from build123d import *

# Parameters (mm, degrees)
ESQUISSE1_R        = 5
ESQUISSE1_R_2      = 2.877506478
ESQUISSE1_R_3      = 3.063484505
ESQUISSE1_R_4      = 2.684325632
ESQUISSE1_R_5      = 0.5
BOSS_EXTRU_1_DEPTH = 3


with BuildPart() as part:
    # Esquisse1 → Boss.-Extru.1 (new body)
    with BuildSketch(Plane.XY):
        with BuildLine():
            Line((6, -6.708203932), (6, 0))
            Line((6, 0), (9, 0))
            Line((9, 0), (9.959071707, 27.096179922))
            ThreePointArc((9.959071707, 27.096179922), (0, 38), (-9.959071707, 27.096179922))
            Line((-9.959071707, 27.096179922), (-9, 0))
            Line((-9, 0), (-6, 0))
            Line((-6, 0), (-6, -6.708203932))
            ThreePointArc((-6, -6.708203932), (0, -9), (6, -6.708203932))
        make_face()
        Circle(ESQUISSE1_R, mode=Mode.SUBTRACT)
        with Locations((-4.874230419, 15.048067775)):
            Circle(ESQUISSE1_R_2, mode=Mode.SUBTRACT)
        with Locations((4.750736526, 13.416152965)):
            Circle(ESQUISSE1_R_3, mode=Mode.SUBTRACT)
        with Locations((-1.177443807, 8.487104148)):
            Circle(ESQUISSE1_R_4, mode=Mode.SUBTRACT)
        with Locations((-7.424621202, 20.575378798)):
            Circle(ESQUISSE1_R_5, mode=Mode.SUBTRACT)
        with Locations((-6.01040764, 21.98959236)):
            Circle(ESQUISSE1_R_5, mode=Mode.SUBTRACT)
        with Locations((0, 36.5)):
            Circle(ESQUISSE1_R_5, mode=Mode.SUBTRACT)
    extrude(amount=BOSS_EXTRU_1_DEPTH)


solid = part.part
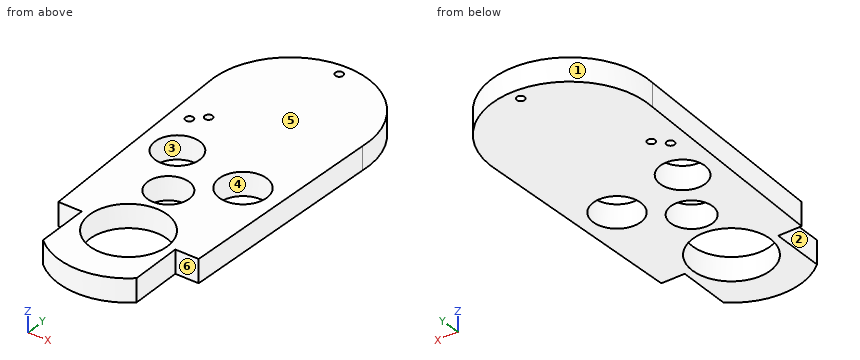
Verification items for the finished model (mm, model axes). Face numbers are marked on the shaded views. A direction names the side the tool comes from. Round coordinates to 2 decimals unless told otherwise and drop trailing zeros. Order: outer loops, then holes, each group sorted by start corner. A loop starts at its lowest first (then second) coordinate and runs counter-clockwise, first axis right, second up.
1. Section check A-A on y = 36.5. Record the cut outline in (x, z), then the cut area to 3 significant figures.
Final values:
outline: (-5.27, 0) - (-0.5, 0) - (-0.5, 3) - (-5.27, 3) - close; (0.5, 0) - (5.27, 0) - (5.27, 3) - (0.5, 3) - close
area: 28.6 mm2
2. Thickness scan on L1, parallel to Y at x = -4.25, z = 1.6; L2, parallel to Y at x = -7, z = 0.7; L3, parallel to X at y = 27, z = 0.3. Record the ranges inside material, lowest first.
Final values:
L1: y = -7.93 to -2.63, 2.63 to 12.24, 17.86 to 37.05
L2: y = 0 to 13.11, 16.99 to 20.31, 20.84 to 35.14
L3: x = -9.96 to 9.96
3. Go/stop test with flat-tipped pins: P1, Ø1.5, axis at y = -4, z = 1, coming from the +X side; P2, Ø3, axis at x = -4, y = 20.5, coming from the -Z side; P3, Ø5, axis at x = -4.87, y = 15.05, coming from the -Z side. Record where each tip stops, or that it passes through.
Final values:
P1: stops at x = 6
P2: stops at z = 0
P3: passes through
4. Section check C-C on z = 2.4. Record the cut outline in (x, y).
Final values:
outline: (-9.96, 27.1) - (-9, 0) - (-6, 0) - (-6, -6.71) arc R9 ccw to (6, -6.71) - (6, 0) - (9, 0) - (9.96, 27.1) arc R10 ccw (long way) to start; hole circle Ø1 at (-7.42, 20.58); hole circle Ø5.76 at (-4.87, 15.05); hole circle Ø1 at (-6.01, 21.99); hole circle Ø10 at (0, 0); hole circle Ø5.37 at (-1.18, 8.49); hole circle Ø1 at (0, 36.5); hole circle Ø6.13 at (4.75, 13.42)
5. Section check D-D on x = 2.75. Record the cut outline in (y, z).
Final values:
outline: (-8.57, 0) - (-4.18, 0) - (-4.18, 3) - (-8.57, 3) - close; (4.18, 0) - (11.1, 0) - (11.1, 3) - (4.18, 3) - close; (15.74, 0) - (37.61, 0) - (37.61, 3) - (15.74, 3) - close
6. Section check B-B on x = -3.25. Record the cut outline in (y, z), then the cut area to 3 significant figures.
Final values:
outline: (-8.39, 0) - (-3.8, 0) - (-3.8, 3) - (-8.39, 3) - close; (3.8, 0) - (6.78, 0) - (6.78, 3) - (3.8, 3) - close; (10.19, 0) - (12.67, 0) - (12.67, 3) - (10.19, 3) - close; (17.42, 0) - (37.46, 0) - (37.46, 3) - (17.42, 3) - close
area: 90.3 mm2
7. Access from +Z, -Z, +X, -X, +Y, -Y to the whole of each face (thin tool, end or side, straight path). Record for the marked faces 5 and 6.
Final values:
face 5: +Z, +X, -X, +Y, -Y
face 6: +Z, -Z, +X, -Y
8. Release check for a two-part mould opening along X. For the marked faces 1, 2, 3 and 4 record: +X half, -X half, draft (parallel to the pull), parting line (faces both ways), or undercut.
Final values:
face 1: parting line
face 2: -X half
face 3: undercut
face 4: undercut
